The listing builds one solid part. Answer for the finished solid, in the listing's coordinates (mm). Face numbers are marked on the shaded views. A direction names the side the tool comes from. Round coordinates to 2 decimals unless told otherwise and drop trailing zeros. Write each loop counter-clockwise with the first axis right and the second up, starting at its lowest first coordinate (ties: lowest second). Pieces come first, ordered by that corner, then holes. Notation, with made-up numbers: M -27,49.5 L -18,49.5 A21 cw -18,74.5 Z; hole C 67,1 d5. An arc over 180 degrees is marked long. Answer as CSV lines item,"result". Start each with the question number.
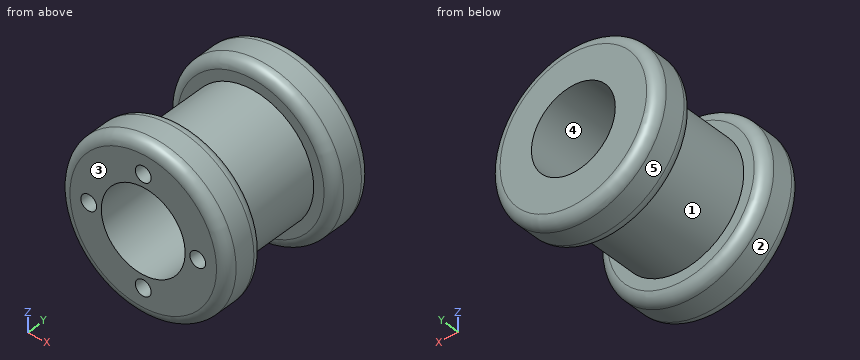
from build123d import *

# Parameters (mm, degrees)
F0_R     = 12.7
F1_DEPTH = 6.35
F2_R     = 9.525
F3_DEPTH = 12.7
F4_R     = 12.7
F5_DEPTH = 6.35
F7_D     = 12.7
F9_D     = 2.3876
F9_DEPTH = 3.175
F9_TIP   = 0.717307407
F10_R    = 1.6002


with BuildPart() as f1:
    # F0 (on Front) → F1 (new body)
    with BuildSketch(Plane.XZ):
        Circle(F0_R)
    extrude(amount=F1_DEPTH)

    # F2 (on face) → F3 (join)
    with BuildSketch(Plane.XZ.offset(6.35)):
        Circle(F2_R)
    extrude(amount=F3_DEPTH)

    # F4 (on face) → F5 (join)
    with BuildSketch(Plane.XZ.offset(19.05)):
        Circle(F4_R)
    extrude(amount=F5_DEPTH)

    # F7 (through all)
    with Locations(Plane.XZ.offset(25.4)):
        with Locations((0, 0)):
            Hole(F7_D / 2)

    # F9
    with Locations(Plane.XZ.offset(25.4)):
        with Locations((0, 8.255), (8.255, 0), (0, -8.255), (-8.255, 0)):
            Hole(F9_D / 2, depth=F9_DEPTH)
            with Locations((0, 0, -(F9_DEPTH + F9_TIP / 2))):  # 118° drill point
                Cone(0, F9_D / 2, F9_TIP, mode=Mode.SUBTRACT)

    # F10
    f10_edges = [f1.edges().sort_by_distance(p)[0] for p in [
        (-12.7, 0, 0),
        (-12.7, -19.05, 0),
        (-12.7, -25.4, 0),
        (-12.7, -6.35, 0),
    ]]
    fillet(f10_edges, radius=F10_R)


solid = f1.part
Q1. For the marked faces 1 and 2, determine the directions among +Z, -Z, +X, -X, +Y, -Y from which every point of the face is accessible in a straight line to the end or side of a thin tool.
Q2. Find section A-A (y = -10.25). Determine the outline of the cut face in (x, z) (3 decimals).
Q3. Straight lines are drawn through the part: L1, parallel to X at y = -13.5, z = -0.25; L2, parallel to Y at x = 10.75, z = -3; L3, parallel to Z at x = -2.5, y = -18.25. For each, find the intervals that lie inside material, in ascending order.
Q4. Each of these flat-tipped pins is pushed along its axis until it touches: P1, Ø6, axis at x = 8, y = -13.5, coming from the -Z side; P2, Ø3, axis at y = -21.5, z = -2.5, coming from the +X side; P3, Ø1.9, axis at x = -8.255, z = 0, coming from the -Y side. Where does it stop, or does it pass through?
Q5. The mould has two halves that part along X. Classify the marked faces 3, 4 and 5: +X half, -X half, draft (parallel to the pull), parting line (faces both ways), or undercut.
Reported:
1,face 1,"none"
1,face 2,"+Y, -Y"
2,outline,"C 0,0 d19.05; hole C 0,0 d12.7"
3,L1,"x = -9.52 to -6.35, 6.35 to 9.52"
3,L2,"y = -25.4 to -19.05, -6.35 to 0"
3,L3,"z = -9.19 to -5.84, 5.84 to 9.19"
4,P1,"stops at z = -8.11"
4,P2,"stops at x = 12.66"
4,P3,"stops at y = -22.08"
5,face 3,"draft"
5,face 4,"undercut"
5,face 5,"parting line"
